Input: part model. Units: mm. Frame: model coordinates. Face numbers are marked on the shaded views. A direction names the side the tool comes from. Round coordinates to 2 decimals unless told otherwise and drop trailing zeros. Loops run counter-clockwise (first coordinate to the right, second up) from the corner with the lowest first, then second, coordinate; pieces in that order, holes last.
(1) Cut plane B-B, the plane z = -12.7. Output: boundary loops of the cut face in (x, y) (1 decimal), and give its area (3 significant figures).
(2) Line query: line 1 (Y direction, x = -15.25, z = 0); line 2 (Z direction, x = -12.25, y = -4) (3 decimals); line 3 (Y direction, x = -15.75, z = 13.5). Output: solid intervals per line, ascending.
(3) First-contact query: pin 1 Ø10.5 at (y, z) = (2.5, 0) entering from +X; pin 2 Ø7 at (y, z) = (2.5, 0) entering from +X; pin 3 Ø4.5 at (x, z) = (-11, -1) entering from -Y. Flat tips, straight axial feed; report the tip coordinate or a pass-through.
(4) Draft query along Y for the marked faces 1, 2 and 3. Return one class per face: released by +Y, released by -Y, zero draft, split by the parting line, or undercut.
(5) Access query for the marked faces 4 and 5. Directions: +Z, -Z, +X, -X, +Y, -Y. A direction counts if a zero-diameter tool reaches every point of the face in a straight line with its end or side. Return the directions, or none.
(6) Cut plane C-C, the plane y = -4. Output: boundary loops of the cut face in (x, z) (1 decimal), and give its area (3 significant figures).
(7) Cut plane D-D, the plane x = -17.5. Output: boundary loops of the cut face in (y, z) (3 decimals), and give its area (3 significant figures).
(8) Cut plane A-A, the plane y = 2.5. Output: boundary loops of the cut face in (x, z) (1 decimal).
from build123d import *

# Parameters (mm, degrees)
F2_DEPTH       = 20
F4_DEPTH       = 6
F6_D           = 3.15
F7_D           = 4.4
F7_CBORE_D     = 8.25
F7_CBORE_DEPTH = 5


with BuildPart() as f2:
    # F1 (on Front) → F2 (new body)
    with BuildSketch(Plane.XZ):
        with BuildLine():
            ThreePointArc((-9.8994949366, -9.8994949366), (-14, 0), (-9.8994949366, 9.8994949366))
            Line((-9.8994949366, 9.8994949366), (-9.8994949366, 14.8994949366))
            Line((-9.8994949366, 14.8994949366), (-21, 18.7))
            Line((-21, 18.7), (-21, -18.7))
            Line((-21, -18.7), (-9.8994949366, -14.8994949366))
            Line((-9.8994949366, -14.8994949366), (-9.8994949366, -9.8994949366))
        make_face()
    extrude(amount=F2_DEPTH)

    # F3 (on face) → F4 (join)
    with BuildSketch(Plane(origin=(0, 0, 0), x_dir=(-1, 0, 0), z_dir=(0, 1, 0))):
        with BuildLine():
            Line((9.8994949366, 14.8994949366), (9.8994949366, 8.4261497732))
            ThreePointArc((9.8994949366, 8.4261497732), (13, 0), (9.8994949366, -8.4261497732))
            Line((9.8994949366, -8.4261497732), (9.8994949366, -14.8994949366))
            Line((9.8994949366, -14.8994949366), (21, -18.7))
            Line((21, -18.7), (21, 18.7))
            Line((21, 18.7), (9.8994949366, 14.8994949366))
        make_face()
    extrude(amount=F4_DEPTH)

    # F6 (through all)
    with Locations(Plane(origin=(-21, 0, 0), x_dir=(0, -1, 0), z_dir=(-1, 0, 0))):
        with Locations((4, 12.7), (4, -12.7)):
            Hole(F6_D / 2)

    # F7 (through all)
    with Locations(Plane(origin=(-21, 0, 0), x_dir=(0, -1, 0), z_dir=(-1, 0, 0))):
        with Locations((-2.5, 0)):
            CounterBoreHole(F7_D / 2, F7_CBORE_D / 2, F7_CBORE_DEPTH)


solid = f2.part
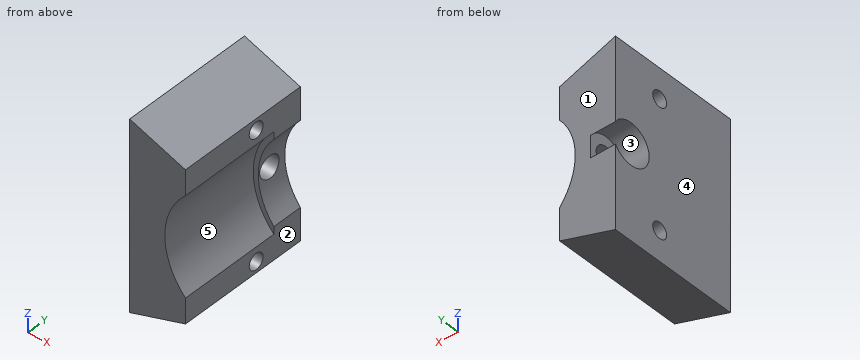
Reported:
1. outline: (-21, -20) - (-9.9, -20) - (-9.9, -5.6) - (-21, -5.6) - close; (-21, -2.4) - (-9.9, -2.4) - (-9.9, 6) - (-21, 6) - close
1. area: 254 mm2
2. line 1: y = -20 to 0.3, 4.7 to 6
2. line 2: z = -15.704 to -14.275, -11.125 to -6.778, 6.778 to 11.125, 14.275 to 15.704
2. line 3: y = -20 to -5.36, -2.64 to 6
3. pin 1: stops at x = -11.89
3. pin 2: stops at x = -12.52
3. pin 3: stops at y = 0
4. face 1: released by +Y
4. face 2: zero draft
4. face 3: undercut
5. face 4: +Z, -Z, -X, +Y, -Y
5. face 5: +X, -Y
6. outline: (-21, -18.7) - (-9.9, -14.9) - (-9.9, -14.3) - (-21, -14.3) - close; (-21, -11.1) - (-9.9, -11.1) - (-9.9, -9.9) arc R14 cw to (-9.9, 9.9) - (-9.9, 11.1) - (-21, 11.1) - close; (-21, 14.3) - (-9.9, 14.3) - (-9.9, 14.9) - (-21, 18.7) - close
6. area: 247 mm2
7. outline: (-20, -17.502) - (6, -17.502) - (6, -2.183) arc R4.125 cw (long way) to (6, 2.183) - (6, 17.502) - (-20, 17.502) - close; hole circle Ø3.15 at (-4, -12.7); hole circle Ø3.15 at (-4, 12.7)
7. area: 843 mm2
8. outline: (-21, -18.7) - (-9.9, -14.9) - (-9.9, -8.4) arc R13 cw to (-12.8, -2.2) - (-16, -2.2) - (-16, -4.1) - (-21, -4.1) - close; (-21, 4.1) - (-16, 4.1) - (-16, 2.2) - (-12.8, 2.2) arc R13 cw to (-9.9, 8.4) - (-9.9, 14.9) - (-21, 18.7) - close
